Could you check a few things on this model? Use its own coordinates, in mm. Coordinates: 2 decimals unless noted, no trailing zeros. Loops run counter-clockwise (first coordinate to the right, second up) from the corner with the lowest first, then second, coordinate; pieces in that order, holes last. Notation, with made-up numbers: (-1, -26.5) - (12, -26.5) arc R29 cw to (12, -6.5) - close; hole circle Ø5 at (53, 3). An arc over 180 degrees is marked (long way). One line per question, with ' | ' between items. Start each with the question number.
1. I'm going to push flat-ended pins straight in: P1, Ø2, axis at y = -61.5, z = 3, coming from the +X side; P2, Ø1.5, axis at x = 40, z = 4, coming from the -Y side; P3, Ø4, axis at x = 20.5, y = -82.72, coming from the +Z side; P4, Ø2, axis at y = -96.5, z = 1.5, coming from the -X side. Where does each tip first touch, or does it pass through?
2. Please list where these lines run through material, in increasing order: L1, parallel to Y at x = 35, z = 1.25; L2, parallel to Y at x = 81, z = 3; L3, parallel to X at y = -13.5, z = 5.5. Write a range as [from, to].
3. We'd pull the mould along X, two halves only. Please class faces 1 (the flat face through (6, -80, 6.35)), 2 (the cylindrical face through (-26.412, -154.325, 3.131)), 3 (the cylindrical face through (20.08, -79.57, 3.22)): pulls with the +X half, pulls with the -X half, needs draft (parallel to the pull), parting line crosses it, or undercut.
4. I want a section at B-B, the plane x = 78.5. Write out the boundary of the cut face in (y, z).
5. I want a section at C-C, the plane y = -127. Write out the boundary of the cut face in (x, z).
Autodesk Inventor part; units mm, degrees
ref_plane "YZ Plane" through (0, 0, 0) normal (1, 0, 0) x (0, 1, 0)
ref_plane "XZ Plane" through (0, 0, 0) normal (0, 1, 0) x (-1, 0, 0)
ref_plane "XY Plane" through (0, 0, 0) normal (0, 0, 1) x (1, 0, 0)
sketch "Sketch1" plane through (0, 0, 0) normal (0, 0, 1) x (1, 0, 0)
  circle A0 centre (-13.8429, -18.2704) radius 12.7
  circle A1 centre (93.4781, -85.2045) radius 12.7
  circle A2 centre (-18.149, -144.6801) radius 12.7
  line L0 (103.5984, -82.1974) -> (-21.5072, -11.0096)
  line L1 (-21.5072, -11.0096) -> (-20.6049, -154.9481)
  line L2 (-20.6049, -154.9481) -> (103.5984, -82.1974)
  point P0 (0, 0)
  point P1 (-21.3977, -28.479)
  point P2 (-1.7779, -22.236)
  point P3 (88.4146, -73.5575)
  point P4 (84.0113, -93.6703)
  point P5 (-20.7472, -132.2488)
  point P6 (-5.5307, -146.1185)
extrude "Extrusion1" add sketch "Sketch1" along normal blind 6.35
sketch "Sketch2" plane through (0, 0, 6.35) normal (0, 0, 1) x (1, 0, 0)
  line L0 (-5.5307, -146.1185) -> (84.0113, -93.6703)
  line L1 (88.4146, -73.5575) -> (-1.7779, -22.236)
  line L2 (-21.3977, -28.479) -> (-20.7472, -132.2488)
  line L3 (43.3184, -47.8967) -> (11.3485, -104.0805) construction
  line L4 (39.2403, -119.8944) -> (11.3485, -72.2762) construction
  line L5 (-21.0724, -80.3639) -> (51.2351, -79.9106) construction
  line L6 (20.479, -80.1034) -> (20.5282, -87.9482) construction
  line L7 (15.9498, -80.1318) -> (22.7682, -84.0116) construction
  line L8 (25.0082, -80.075) -> (18.239, -84.04) construction
  circle A0 centre (20.4954, -82.7183) radius 3.175
  point P0 (0, 0)
  dimension "d2" = 6.35
extrude "Extrusion2" cut sketch "Sketch2" against normal through all
properties part number "motorPlate" material "Aluminum 6061"
Results are:
1) P1: stops at x = 68.98 | P2: stops at y = -119.89 | P3: passes through | P4: stops at x = -20.98
2) L1: y = [-122.38, -43.16] | L2: y = [-95.43, -69.34] | L3: x = [-25.61, -2.07]
3) face 1: needs draft | face 2: parting line crosses it | face 3: undercut
4) outline: (-96.9, 0) - (-67.92, 0) - (-67.92, 6.35) - (-96.9, 6.35) - close
5) outline: (-20.78, 0) - (27.11, 0) - (27.11, 6.35) - (-20.78, 6.35) - close
